Build history of the part. All positions in model axes, mm. Coordinates: 2 decimals unless noted, no trailing zeros. Order: outer loops, then holes, each group sorted by start corner. A loop starts at its lowest first (then second) coordinate and runs counter-clockwise, first axis right, second up. Notation, with made-up numbers: (-24, 9.25) - (-20, 9.25) arc R33 cw to (-20, 46.25) - close; hole circle Ø7 at (53, 49). An arc over 180 degrees is marked (long way). Write each question's results on one line, items separated by ' | '.
from build123d import *

# Parameters (mm, degrees)
SKETCH1_R           = 1.1557
BOSS_EXTRUDE1_DEPTH = 0.7366
SKETCH2_R           = 1.651
SKETCH2_R_2         = 1.1557
BOSS_EXTRUDE2_DEPTH = 3.175


with BuildPart() as part:
    # Sketch1 → Boss-Extrude1 (new body)
    with BuildSketch(Plane(origin=(0, 0, 0), x_dir=(0, 0, -1), z_dir=(1, 0, 0))):
        with BuildLine():
            ThreePointArc((1.5875, 2.482159687), (-2.9464, 0), (1.5875, -2.482159687))
            ThreePointArc((1.5875, -2.482159687), (3.175, -2.017919373), (4.7625, -2.482159687))
            ThreePointArc((4.7625, -2.482159687), (9.2964, 0), (4.7625, 2.482159687))
            ThreePointArc((4.7625, 2.482159687), (3.175, 2.017919373), (1.5875, 2.482159687))
        make_face()
        Circle(SKETCH1_R, mode=Mode.SUBTRACT)
        with Locations((6.35, 0)):
            Circle(SKETCH1_R, mode=Mode.SUBTRACT)
    boss_extrude1 = extrude(amount=BOSS_EXTRUDE1_DEPTH)

    # Sketch2 → Boss-Extrude2 (add)
    # profile 1 of 2: a face of its own
    with BuildSketch(Plane(origin=(0.7366, 0, 0), x_dir=(0, 0, -1), z_dir=(1, 0, 0))):
        Circle(SKETCH2_R)
        Circle(SKETCH2_R_2, mode=Mode.SUBTRACT)
    # profile 2 of 2: a face of its own
    with BuildSketch(Plane(origin=(0.7366, 0, 0), x_dir=(0, 0, -1), z_dir=(1, 0, 0))):
        with Locations((6.35, 0)):
            Circle(SKETCH2_R)
        with Locations((6.35, 0)):
            Circle(SKETCH2_R_2, mode=Mode.SUBTRACT)
    extrude(amount=BOSS_EXTRUDE2_DEPTH)

    # Mirror1: Boss-Extrude1 across plane
    add(boss_extrude1.mirror(Plane(origin=(2.3241, 0, 0), x_dir=(0, 0, 1), z_dir=(1, 0, 0))))


solid = part.part
1. Band-saw the part on C-C on z = 0. Give the cut face in (x, y).
Solved:
outline: (0, -2.95) - (0.74, -2.95) - (0.74, -1.65) - (3.91, -1.65) - (3.91, -2.95) - (4.65, -2.95) - (4.65, -1.16) - (0, -1.16) - close; (0, 1.16) - (4.65, 1.16) - (4.65, 2.95) - (3.91, 2.95) - (3.91, 1.65) - (0.74, 1.65) - (0.74, 2.95) - (0, 2.95) - close
2. Band-saw the part on B-B on x = 1. Give the cut face in (y, z).
Solved:
outline: circle Ø3.3 at (0, -6.35); circle Ø3.3 at (0, 0); hole circle Ø2.31 at (0, -6.35); hole circle Ø2.31 at (0, 0)
3. Two-plate mould, pull along X, no slides. Class faces 1 (the face through (0, 0, -3)), 2 (the face through (0.737, 0, -3)), 3 (the face through (4.648, 0, -3)), 4 (the face through (3.912, 0, -3)): +X half, -X half, draft (parallel to the pull), parting line (faces both ways), or undercut.
Solved:
face 1: -X half | face 2: undercut | face 3: +X half | face 4: undercut
4. Band-saw the part on A-A on y = 0. Give the cut face in (x, z).
Solved:
outline: (0, -9.3) - (0.74, -9.3) - (0.74, -8) - (3.91, -8) - (3.91, -9.3) - (4.65, -9.3) - (4.65, -7.51) - (0, -7.51) - close; (0, -5.19) - (4.65, -5.19) - (4.65, -1.16) - (0, -1.16) - close; (0, 1.16) - (4.65, 1.16) - (4.65, 2.95) - (3.91, 2.95) - (3.91, 1.65) - (0.74, 1.65) - (0.74, 2.95) - (0, 2.95) - close; hole (0.74, -4.7) - (3.91, -4.7) - (3.91, -1.65) - (0.74, -1.65) - close
5. Probe line 1 (X direction, y = 1.6, z = -0.75); line 2 (Y direction, x = 2.75, z = -6.35); line 3 (Y direction, x = 4.2, z = -6.35). List the from-to ranges inside material, lowest first.
Solved:
line 1: x = 0 to 0.74, 3.91 to 4.65 | line 2: y = -1.65 to -1.16, 1.16 to 1.65 | line 3: y = -2.95 to -1.16, 1.16 to 2.95
6. Band-saw the part on D-D on y = 2.2. Give the cut face in (x, z).
Solved:
outline: (0, -8.31) - (0.74, -8.31) - (0.74, -4.19) - (0, -4.19) - close; (0, -2.16) - (0.74, -2.16) - (0.74, 1.96) - (0, 1.96) - close; (3.91, -8.31) - (4.65, -8.31) - (4.65, -4.19) - (3.91, -4.19) - close; (3.91, -2.16) - (4.65, -2.16) - (4.65, 1.96) - (3.91, 1.96) - close
